from build123d import *

# Parameters (mm, degrees)
SKETCH_1_W               = 26
SKETCH_1_H               = 11
SKETCH_1_R               = 1
EXTRUDE_1_DEPTH          = 2
SKETCH_2_R               = 3.315
EXTRUDE_2_DEPTH          = 26
FILLET_1_R               = 10
CUT_EXTRUDE_1_DEPTH      = 18.748239349
CUT_EXTRUDE_1_DEPTH_BACK = 18.748239349
SKETCH_3_W               = 8
SKETCH_3_H               = 6.63


with BuildPart() as part:
    # 草图1 → 凸台-拉伸1 (new body)
    with BuildSketch(Plane(origin=(0, 0, 0), x_dir=(1, 0, 0), z_dir=(0, 1, 0))):
        with Locations((0, -5.5)):
            Rectangle(SKETCH_1_W, SKETCH_1_H)
        with Locations(Location((9, -7.5, 0), (0, 0, 270))):
            Circle(SKETCH_1_R, mode=Mode.SUBTRACT)
        with Locations(Location((-9, -7.5, 0), (0, 0, 90))):
            Circle(SKETCH_1_R, mode=Mode.SUBTRACT)
    extrude(amount=EXTRUDE_1_DEPTH)

    # 草图2 → 凸台-拉伸2 (add)
    with BuildSketch(Plane(origin=(13, 0, 0), x_dir=(0, 0, -1), z_dir=(1, 0, 0))):
        with Locations((0, 3.685)):
            Circle(SKETCH_2_R)
    extrude(amount=-EXTRUDE_2_DEPTH)

    # 圆角1
    # the kernel refuses this fillet: 10 mm, written as the material it takes off along each edge
    with BuildSketch(Plane(origin=(19.737534787, 0, 0), x_dir=(0, 1, 0), z_dir=(-1, 0, 0))) as fillet_1_piece_1:
        with BuildLine():
            CenterArc((10, -2.695013915), FILLET_1_R, 164.365401099, 15.634598901)
            Line((0, -2.695013915), (-0.2, -2.695013915))
            Line((-0.2, -2.695013915), (-0.2, 0))
            Line((-0.2, 0), (0, 0.2))
            ThreePointArc((0, 0.2), (0.185, 0.2), (0.1774, 0.053900278))
            Line((0.1774, 0.053900278), (0.37, 0))
        make_face()
    extrude(amount=39.475069573, mode=Mode.SUBTRACT)

    # 草图3 → 切除-拉伸1 (cut, two sides: drawn at the far end of the back side and taken through both)
    with BuildSketch(Plane(origin=(0, 2, 0), x_dir=(1, 0, 0), z_dir=(0, 1, 0)).offset(-CUT_EXTRUDE_1_DEPTH_BACK)):
        with Locations((9, 0)):
            Rectangle(SKETCH_3_W, SKETCH_3_H)
        with Locations((-9, 0)):
            Rectangle(SKETCH_3_W, SKETCH_3_H)
    extrude(amount=CUT_EXTRUDE_1_DEPTH + CUT_EXTRUDE_1_DEPTH_BACK, mode=Mode.SUBTRACT)


solid = part.part
For this review, take the finished solid that the model builds, in its own axes (mm). A direction names the side the tool comes from. Coordinates: 2 decimals unless noted, no trailing zeros. Write each loop counter-clockwise with the first axis right and the second up, starting at its lowest first coordinate (ties: lowest second). Pieces come first, ordered by that corner, then holes. Notation, with made-up numbers: (-29, 5) -> (3, 5) arc R19 cw to (3, 31) -> close; hole circle Ø7 at (25.5, -15.5). An arc over 180 degrees is marked (long way). Write each question's results on one line, items separated by ' | '. Start each with the question number.
1) Consider section A-A (z = 7.5). Write out the cut boundary in (x, y).
2) Consider section D-D (z = 5.25). Write out the cut boundary in (x, y).
3) Consider section B-B (x = -9). Write out the cut boundary in (y, z) (3 decimals).
4) Wall thickness on L1, parallel to X at y = 0.4, z = 7.5; L2, parallel to Y at x = 10.25, z = 6.25; L3, parallel to Z at x = -10.5, y = 0.5 (3 decimals): over which ranges is each line inside the solid? List them lowest first. Write a range as [from, to].
5) Consider section C-C (x = 11.5). Write out the cut boundary in (y, z) (3 decimals), plus the area to 3 significant figures.
6) The part is to be moulded in two halves that separate along X. For faces 1 (the face through (-9, 1, 3.315)), 2 (the face through (9.99, 0.99, 7.37)), 3 (the face through (5, 3, 0)), say which applies: +X half, -X half, draft (parallel to the pull), parting line (faces both ways), or undercut.
7) For faces 4 (the face through (9, 1, 3.315)), 5 (the face through (13, 1, 7)), 6 (the face through (-5, 3, 0)), list the 3-axis set-ups (+Z, -Z, +X, -X, +Y, -Y) from which the entire face can be reached by the end or side of a thin tool; tool diameter is ignored.
8) Insertion check: pin 1 (1 mm diameter, centred on y = 4, z = 8, fed in from -X); pin 2 (3 mm diameter, centred on x = -9, z = 7.5, fed in from +Y); pin 3 (2 mm diameter, centred on y = 2, z = 0.5, fed in from -X); pin 4 (2 mm diameter, centred on y = 3, z = 3, fed in from +X). Each pin has a flat end and moves straight along its axis. Give the tip position at first contact, or say it passes through.
Geometry says:
1) outline: (-13, 0) -> (-10, 0) -> (-10, 2) -> (-13, 2) -> close; (-8, 0) -> (8, 0) -> (8, 2) -> (-8, 2) -> close; (10, 0) -> (13, 0) -> (13, 2) -> (10, 2) -> close
2) outline: (-13, 0) -> (13, 0) -> (13, 2) -> (-13, 2) -> close
3) outline: (0, 3.315) -> (2, 3.315) -> (2, 6.5) -> (0, 6.5) -> close; (0, 8.5) -> (2, 8.5) -> (2, 11) -> (0, 11) -> close
4) L1: [-13, -10], [-8, 8], [10, 13] | L2: [0, 2] | L3: [3.315, 11]
5) outline: (0, 3.315) -> (2, 3.315) -> (2, 11) -> (0, 11) -> close | area: 15.4 mm^2
6) face 1: draft | face 2: undercut | face 3: +X half
7) face 4: -Z, +X, +Y, -Y | face 5: +Z, -Z, +X, +Y, -Y | face 6: -Z, -X, +Y, -Y
8) pin 1: through | pin 2: y = 2 | pin 3: x = -5 | pin 4: x = 5
